Verification items for the finished model (mm, model axes). A direction names the side the tool comes from. Coordinates: 2 decimals unless noted, no trailing zeros. Order: outer loops, then holes, each group sorted by start corner. A loop starts at its lowest first (then second) coordinate and runs counter-clockwise, first axis right, second up. Notation, with made-up numbers: M 26.5,80 L 59.5,80 A28 cw 59.5,104 Z; hole C 19,7.25 d2. An arc over 180 degrees is marked long. Return JSON: item names as keys, results as strings. Group by question number.
1. Material ranges on line 1 along Y through (x, z) = (12.25, 298.45) (3 decimals); line 2 along Y through (x, z) = (5, 406.4) (3 decimals); line 3 along Z through (x, y) = (11.25, -307) (3 decimals), recorded low to high.
2. Section check C-C, the plane z = 174.5. Record the cut outline in (x, y) (3 decimals).
3. Set-up check for faces 1 (the flat face through (19.05, -204, 1161)), 2 (the cylindrical face through (9.4, -330.3, 133.6)): record each of +Z, -Z, +X, -X, +Y, -Y from which the full face is reachable in a straight line by a thin tool's end or side.
4. Mould release check, pull along Z, two halves, no side actions. Record for faces 3 (the cylindrical face through (9.39, -303.61, 161.4)), 4 (the flat face through (0, -204, 1161)): +Z half, -Z half, draft (parallel to the pull), parting line (faces both ways), or undercut.
5. Section check B-B, the plane x = 6. Record the cut outline in (y, z) (3 decimals).
```python
from build123d import *

# Parameters (mm, degrees)
F0_W     = 403.225
F0_H     = 2289.175
F0_R     = 6.35
F1_DEPTH = 19.05
F2_D     = 25.4


with BuildPart() as f1:
    # F0 (on Right) → F1 (new body)
    with BuildSketch(Plane.YZ):
        with Locations((-201.6125, 1144.5875)):
            Rectangle(F0_W, F0_H)
        with Locations((-304.8, 406.4)):
            Circle(F0_R, mode=Mode.SUBTRACT)
        with BuildLine():
            Line((-383.2982277284, 344.7619689838), (-345.7770523386, 338.1459734147))
            ThreePointArc((-345.7770523386, 338.1459734147), (-302.0105735906, 159.2871373286), (-140.5738027921, 70.7198920162))
            Line((-140.5738027921, 70.7198920162), (-143.8944365908, 32.7648740189))
            ThreePointArc((-143.8944365908, 32.7648740189), (-332.2373358557, 136.0933268834), (-383.2982277284, 344.7619689838))
        make_face(mode=Mode.SUBTRACT)
    extrude(amount=F1_DEPTH)

    # F2 (through all)
    with Locations(Plane(origin=(0, 0, 0), x_dir=(0, 1, 0), z_dir=(-1, 0, 0))):
        with Locations((-120.65, -298.45)):
            Hole(F2_D / 2)


solid = f1.part
```
Answers follow:
{
 "1": {"line 1": "-403.225 to -387.35, -349.25 to -133.35, -107.95 to 0", "line 2": "-403.225 to -311.15, -298.45 to 0", "line 3": "0 to 107.655, 166.043 to 400.443, 412.357 to 2289.175"},
 "2": {"outline": "M 0,-403.225 L 19.05,-403.225 L 19.05,-356.797 L 0,-356.797 Z; M 0,-312.729 L 19.05,-312.729 L 19.05,0 L 0,0 Z"},
 "3": {"face 1": "+Z, -Z, +X, +Y, -Y", "face 2": "+X, -X"},
 "4": {"face 3": "undercut", "face 4": "draft"},
 "5": {"outline": "M -403.225,0 L 0,0 L 0,2289.175 L -403.225,2289.175 Z; hole M -383.298,344.762 A266.7 ccw -143.894,32.765 L -140.574,70.72 A228.6 cw -345.777,338.146 Z; hole C -304.8,406.4 d12.7; hole C -120.65,298.45 d25.4"}
}
